from build123d import *

# Parameters (mm, degrees)
SKETCH1_R           = 50.8
BOSS_EXTRUDE1_DEPTH = 38.1
REVOLVE1_ANGLE      = 180
BOSS_EXTRUDE2_DEPTH = 203.2
SKETCH5_W           = 76.2
SKETCH5_H           = 279.4
CUT_EXTRUDE1_DEPTH  = 12.7
SKETCH6_R           = 19.704792108
BOSS_EXTRUDE3_DEPTH = 101.6
SKETCH7_R           = 6.35
BOSS_EXTRUDE4_DEPTH = 50.8
SKETCH8_R           = 12.7
BOSS_EXTRUDE5_DEPTH = 25.4
CUT_EXTRUDE2_DEPTH  = 12.7


with BuildPart() as part:
    # Sketch1 → Boss-Extrude1 (new body)
    with BuildSketch(Plane.XY):
        with Locations(Location((0, 0, 0), (0, 0, 180))):
            Circle(SKETCH1_R)
    extrude(amount=BOSS_EXTRUDE1_DEPTH)

    # Sketch2 → Revolve1 (revolve)
    with BuildSketch(Plane.XY.offset(38.1)):
        with BuildLine():
            Line((0, 76.2), (0, -76.2))
            ThreePointArc((0, -76.2), (76.2, 0), (0, 76.2))
        make_face()
    revolve(axis=Axis((0, 76.2, 38.1), (0, -1, 0)), revolution_arc=REVOLVE1_ANGLE)

    # Sketch3 → Boss-Extrude2 (add)
    with BuildSketch(Plane(origin=(0, 0, 0), x_dir=(1, 0, 0), z_dir=(0, 1, 0))):
        with BuildLine():
            Line((-76.2, -38.1), (76.2, -38.1))
            ThreePointArc((76.2, -38.1), (0, -114.3), (-76.2, -38.1))
        make_face()
    extrude(amount=-BOSS_EXTRUDE2_DEPTH)

    # Sketch5 → Cut-Extrude1 (cut)
    with BuildSketch(Plane(origin=(76.2, 0, 0), x_dir=(0, 0, -1), z_dir=(1, 0, 0))):
        with Locations((-76.2, -63.5)):
            Rectangle(SKETCH5_W, SKETCH5_H)
    cut_extrude1 = extrude(amount=-CUT_EXTRUDE1_DEPTH, mode=Mode.SUBTRACT)

    # Mirror1: Cut-Extrude1 across plane
    add(cut_extrude1.mirror(Plane(origin=(0, 0, 0), x_dir=(0, 0, 1), z_dir=(1, 0, 0))), mode=Mode.SUBTRACT)

    # Sketch6 → Boss-Extrude3 (add)
    with BuildSketch(Plane(origin=(0, 0, 0), x_dir=(-1, 0, 0), z_dir=(0, 0, -1))):
        Circle(SKETCH6_R)
    extrude(amount=BOSS_EXTRUDE3_DEPTH)

    # Sketch7 → Boss-Extrude4 (add)
    with BuildSketch(Plane.XZ.offset(203.2)):
        with Locations(Location((0, 76.2, 0), (0, 0, 270))):
            Circle(SKETCH7_R)
    extrude(amount=BOSS_EXTRUDE4_DEPTH)

    # Sketch8 → Boss-Extrude5 (add)
    with BuildSketch(Plane.XZ.offset(254)):
        with Locations(Location((0, 76.2, 0), (0, 0, 270))):
            Circle(SKETCH8_R)
    extrude(amount=BOSS_EXTRUDE5_DEPTH)

    # Sketch9 → Cut-Extrude2 (cut)
    with BuildSketch(Plane.XZ.offset(279.4)):
        with BuildLine():
            Line((0, 83.631744278), (0, 85.853587437))
            ThreePointArc((0, 85.853587437), (-4.437705251, 84.773127931), (-7.882046977, 81.773606182))
            Line((-7.882046977, 81.773606182), (-6.067936702, 80.490800298))
            ThreePointArc((-6.067936702, 80.490800298), (-3.416335204, 82.799960363), (0, 83.631744278))
        make_face()
        with BuildLine():
            Line((6.067936702, 80.490800298), (7.882046977, 81.773606182))
            ThreePointArc((7.882046977, 81.773606182), (9.608703215, 77.129824142), (8.804494423, 72.241132945))
            Line((8.804494423, 72.241132945), (6.778076179, 73.152294908))
            ThreePointArc((6.778076179, 73.152294908), (7.397190485, 76.915818372), (6.067936702, 80.490800298))
        make_face()
        with BuildLine():
            Line((-6.778076179, 73.152294908), (-8.804494423, 72.241132945))
            ThreePointArc((-8.804494423, 72.241132945), (-5.242827536, 68.094168159), (0, 66.546412563))
            Line((0, 66.546412563), (0, 68.768255722))
            ThreePointArc((0, 68.768255722), (-4.036152756, 69.959784142), (-6.778076179, 73.152294908))
        make_face()
    extrude(amount=-CUT_EXTRUDE2_DEPTH, mode=Mode.SUBTRACT)


solid = part.part
Verification items for the finished model (mm, model axes). A direction names the side the tool comes from. Coordinates: 2 decimals unless noted, no trailing zeros. Write each loop counter-clockwise with the first axis right and the second up, starting at its lowest first coordinate (ties: lowest second). Pieces come first, ordered by that corner, then holes. Notation, with made-up numbers: (86.25, 86) -> (113.25, 86) arc R6 ccw to (113.25, 90) -> close; hole circle Ø9 at (-6, 78). An arc over 180 degrees is marked (long way). One line per item, written item: value. Start each with the question number.
Q1. Access from +Z, -Z, +X, -X, +Y, -Y to the whole of each face (thin tool, end or side, straight path). Record for faces 4 (the flat face through (0, -279.4, 76)), 5 (the cylindrical face through (-23.44, 45.07, 18.78)), 6 (the flat face through (-3, -254, 82)), 7 (the cylindrical face through (9.6, -273.1, 77.2)), 8 (the flat face through (-63.5, -79, 59)).
Q2. Cross-section at C-C on x = 55. Enter the section's corners in (y, z).
Q3. Go/stop test with flat-tipped pins: P1, Ø10, axis at y = -4, z = -69, coming from the -X side; P2, Ø4.5, axis at x = -5, z = 84, coming from the -Y side; P3, Ø20.5, axis at x = -5, z = 80.5, coming from the +Y side; P4, Ø10, axis at x = -18, y = 40, coming from the +Z side. Record where each tip stops, or that it passes through.
Q4. Thickness scan on L1, parallel to Z at x = -3, y = -99; L2, parallel to Y at x = -8.5, z = -28; L3, parallel to Z at x = -36, y = -11. Record the ranges inside material, lowest first. Write a range as from..to.
Q5. Mould release check, pull along X, two halves, no side actions. Record for faces 1 (the cylindrical face through (-4.38, -273.139, 84.803)), 2 (the cylindrical face through (1.051, -100.178, 114.293)), 3 (the flat face through (1, -203.2, 67)): pulls with the +X half, pulls with the -X half, needs draft (parallel to the pull), parting line crosses it, or undercut.
Q6. Cross-section at B-B on y = -26. Enter the section's corners in (x, z).
Q7. Cross-section at D-D on y = -210. Enter the section's corners in (x, z), and give its area (3 significant figures).
Q8. Cross-section at A-A on z = 16. Enter the section's corners in (x, y).
Checked values:
1. face 4: +Z, -Z, +X, -X, -Y
1. face 5: -Z
1. face 6: none
1. face 7: -Y
1. face 8: +Z, -Z, -X, +Y, -Y
2. outline: (-203.2, 38.1) -> (52.74, 38.1) arc R52.74 ccw to (0, 90.84) -> (-203.2, 90.84) -> close
3. P1: stops at x = -19.7
3. P2: stops at y = -279.4
3. P3: stops at y = 68.95
3. P4: stops at z = 103.64
4. L1: z = 38.1..114.24
4. L2: y = -17.78..17.78
4. L3: z = 0..105.26
5. face 1: undercut
5. face 2: parting line crosses it
5. face 3: needs draft
6. outline: (-63.5, 38.1) -> (-43.64, 38.1) -> (-43.64, 0) -> (43.64, 0) -> (43.64, 38.1) -> (63.5, 38.1) -> (63.5, 80.22) arc R76.2 ccw to (-63.5, 80.22) -> close
7. outline: circle Ø12.7 at (0, 76.2)
7. area: 127 mm²
8. outline: circle Ø101.6 at (0, 0)
